The model under review builds one solid part; all positions refer to its coordinate system, in mm. A direction names the side the tool comes from. Coordinates: 2 decimals unless noted, no trailing zeros. Order: outer loops, then holes, each group sorted by start corner. A loop starts at its lowest first (then second) coordinate and runs counter-clockwise, first axis right, second up.
from build123d import *

# Parameters (mm, degrees)
SKETCH1_W           = 52
SKETCH1_H           = 38
BOSS_EXTRUDE1_DEPTH = 7.6
SKETCH2_R           = 2
BOSS_EXTRUDE2_DEPTH = 48
BOSS_EXTRUDE3_DEPTH = 5


with BuildPart() as part:
    # Sketch1 → Boss-Extrude1 (new body)
    with BuildSketch(Plane(origin=(0, 0, 0), x_dir=(1, 0, 0), z_dir=(0, 1, 0))):
        with Locations((-14.781119537, 0)):
            Rectangle(SKETCH1_W, SKETCH1_H)
    extrude(amount=BOSS_EXTRUDE1_DEPTH)

    # Sketch2 → Boss-Extrude2 (add)
    with BuildSketch(Plane(origin=(11.218880463, 0, 0), x_dir=(0, 0, -1), z_dir=(1, 0, 0))):
        with Locations(Location((-14.368237461, 3.8, 0), (0, 0, 180))):
            Circle(SKETCH2_R)
    extrude(amount=BOSS_EXTRUDE2_DEPTH)

    # Sketch3 → Boss-Extrude3 (add)
    with BuildSketch(Plane(origin=(59.218880463, 0, 0), x_dir=(0, 0, -1), z_dir=(1, 0, 0))):
        Polygon((-16.050594412, 2.718484817), (-12.685880511, 2.718484817), (-14.368237461, 22.718484817), align=None)
    extrude(amount=BOSS_EXTRUDE3_DEPTH)


solid = part.part
(1) Consider section C-C (z = -7). Give the boundary of the cut face in (x, y), then the cut area to 3 significant figures.
(2) Consider section A-A (x = 23.5). Give the boundary of the cut face in (y, z).
(3) Insertion check: pin 1 Ø11.5 at (x, z) = (-10, -4.5) entering from +Y; pin 2 Ø4 at (y, z) = (3, 1.5) entering from +X; pin 3 Ø1.7 at (x, z) = (62, 14.5) entering from -Y. Each pin has a flat end and moves straight along its axis. Give the tip position at first contact, or say it passes through.
(4) Consider section B-B (y = 3.8). Give the boundary of the cut face in (x, z), then the cut area to 3 significant figures.
(5) Consider section D-D (x = -26.5). Give the boundary of the cut face in (y, z), then the cut area to 3 significant figures.
(6) Wall thickness on line 1 (Y direction, x = -14, z = 4); line 2 (X direction, y = 2.5, z = -9); line 3 (Z direction, x = 20, y = 2.75): over which ranges is each line inside the solid? List them lowest first.
(7) The part is to be moulded in two halves that separate along X. For faces 1 (the face through (64.219, 11, 14)), 2 (the face through (34.88, 2.45, 12.89)), 3 (the face through (59.219, 12, 14)), 4 (the face through (62, 2.718, 14)), say which applies: +X half, -X half, draft (parallel to the pull), parting line (faces both ways), or undercut.
(8) Tool access review of faces 5 (the face through (61.684, 12.578, 13.515)), 6 (the face through (61.684, 12.858, 15.198)), 7 (the face through (-15, 0, 0)): name each direction out of +Z, -Z, +X, -X, +Y, -Y from which nothing blocks a thin tool from reaching the whole face with its end or side.
Findings:
1. outline: (-40.78, 0) - (11.22, 0) - (11.22, 7.6) - (-40.78, 7.6) - close
1. area: 395 mm2
2. outline: circle Ø4 at (3.8, 14.37)
3. pin 1: stops at y = 7.6
3. pin 2: stops at x = 11.22
3. pin 3: stops at y = 2.72
4. outline: (-40.78, -19) - (11.22, -19) - (11.22, 12.37) - (59.22, 12.37) - (59.22, 12.78) - (64.22, 12.78) - (64.22, 15.96) - (59.22, 15.96) - (59.22, 16.37) - (11.22, 16.37) - (11.22, 19) - (-40.78, 19) - close
4. area: 2,180 mm2
5. outline: (0, -19) - (7.6, -19) - (7.6, 19) - (0, 19) - close
5. area: 289 mm2
6. line 1: y = 0 to 7.6
6. line 2: x = -40.78 to 11.22
6. line 3: z = 12.67 to 16.07
7. face 1: +X half
7. face 2: undercut
7. face 3: undercut
7. face 4: draft
8. face 5: -Z, +X, +Y
8. face 6: +Z, +X, +Y
8. face 7: +Z, -Z, +X, -X, -Y
